The listing builds one solid part. Answer for the finished solid, in the listing's coordinates (mm). A direction names the side the tool comes from. Give positions to 0.01 mm unless a question says otherwise; leave off trailing zeros. Order: outer loops, then holes, each group sorted by start corner. A loop starts at its lowest first (then second) coordinate and runs counter-clockwise, first axis right, second up.
```python
from build123d import *

# Parameters (mm, degrees)
EXTRUDE_1_DEPTH = 4.2
SKETCH_2_R      = 3.5
EXTRUDE_2_DEPTH = 2.1
SKETCH_3_R      = 2.25
EXTRUDE_3_DEPTH = 2
EXTRUDE_START   = -9
EXTRUDE_4_DEPTH = 7


with BuildPart() as part:
    # 草图1 → 凸台-拉伸1 (new body)
    with BuildSketch(Plane.XY):
        with BuildLine():
            ThreePointArc((-6.25, 3.3e-08), (-5.817755734, -2.236089463), (-4.583301282, -4.15))
            Line((-4.583301282, -4.15), (4.583301282, -4.15))
            ThreePointArc((4.583301282, -4.15), (5.817755724, -2.236089488), (6.25, -2.1e-08))
            ThreePointArc((6.25, -2.1e-08), (5.817755732, 2.236089469), (4.583301282, 4.15))
            Line((4.583301282, 4.15), (-4.583301282, 4.15))
            ThreePointArc((-4.583301282, 4.15), (-5.817755722, 2.236089494), (-6.25, 3.3e-08))
        make_face()
    extrude(amount=EXTRUDE_1_DEPTH)

    # 草图2 → 凸台-拉伸2 (add)
    with BuildSketch(Plane.XY.offset(4.2)):
        Circle(SKETCH_2_R)
    extrude(amount=EXTRUDE_2_DEPTH)

    # 草图3 → 凸台-拉伸3 (add)
    with BuildSketch(Plane.XY.offset(6.3)):
        Circle(SKETCH_3_R)
    extrude(amount=EXTRUDE_3_DEPTH)

    # 草图4 → 凸台-拉伸4 (add)
    with BuildSketch(Plane.XY.offset(4.2).offset(EXTRUDE_START)):
        with BuildLine():
            ThreePointArc((-5.812148865, -2.25), (-6.25, 0), (-5.812148865, 2.25))
            Line((-5.812148865, 2.25), (-7, 2.25))
            Line((-7, 2.25), (-7, -2.25))
            Line((-7, -2.25), (-5.812148865, -2.25))
        make_face()
        with BuildLine():
            Line((7, 2.25), (5.812148865, 2.25))
            ThreePointArc((5.812148865, 2.25), (6.25, 0), (5.812148865, -2.25))
            Line((5.812148865, -2.25), (7, -2.25))
            Line((7, -2.25), (7, 2.25))
        make_face()
    extrude(amount=EXTRUDE_4_DEPTH)


solid = part.part
```
1) Find section B-B (x = 0). Write down the section's boundary in (y, z), then the cut area to 3 significant figures.
Geometry says:
outline: (-4.15, 0) - (4.15, 0) - (4.15, 4.2) - (3.5, 4.2) - (3.5, 6.3) - (2.25, 6.3) - (2.25, 8.3) - (-2.25, 8.3) - (-2.25, 6.3) - (-3.5, 6.3) - (-3.5, 4.2) - (-4.15, 4.2) - close
area: 58.6 mm2
2) Find section D-D (z = 4.5). Write down the section's boundary in (x, y).
Geometry says:
outline: circle Ø7 at (0, 0)
3) Straight lines are drawn through the part: probe 1 along Z at (x, y) = (2.75, 2.5); probe 2 along Z at (x, y) = (1, -3.25); probe 3 along X at (y, z) = (0.5, -2.75). For each, find the intervals that lie inside material, in ascending order.
Geometry says:
probe 1: z = 0 to 4.2
probe 2: z = 0 to 6.3
probe 3: x = -7 to -6.23, 6.23 to 7
4) A tool of negligible diameter and unlimited length cuts with its end or side. For faces 5 (the flat face through (-6, -2.25, -1)), 6 (the flat face through (-6, 2.25, -1)), 7 (the flat face through (0, -4, 4.2)), 8 (the flat face through (6, -2.25, -1)), 9 (the cylindrical face through (-6.25, -0.03, -2.43)), from which of +Z, -Z, +X, -X, +Y, -Y can it reach the whole face along a straight path? Write none if from no direction.
Geometry says:
face 5: +Z, -Z, -X, -Y
face 6: +Z, -Z, -X, +Y
face 7: +Z
face 8: +Z, -Z, +X, -Y
face 9: -Z
5) Find section C-C (y = -1.25). Write down the section's boundary in (x, z).
Geometry says:
outline: (-7, -4.8) - (-6.12, -4.8) - (-6.12, 0) - (6.12, 0) - (6.12, -4.8) - (7, -4.8) - (7, 2.2) - (6.12, 2.2) - (6.12, 4.2) - (3.27, 4.2) - (3.27, 6.3) - (1.87, 6.3) - (1.87, 8.3) - (-1.87, 8.3) - (-1.87, 6.3) - (-3.27, 6.3) - (-3.27, 4.2) - (-6.12, 4.2) - (-6.12, 2.2) - (-7, 2.2) - close
6) For a pull along Y with two mould halves and no side action, classify faces 1 (the flat face through (7, 0, -1)), 2 (the cylindrical face through (6.25, 0.03, -2.43)), 3 (the flat face through (6, 2.25, -1)), 4 (the cylindrical face through (3.233, -1.341, 5.235)) as +Y half, -Y half, draft (parallel to the pull), parting line (faces both ways), or undercut.
Geometry says:
face 1: draft
face 2: undercut
face 3: +Y half
face 4: parting line
7) Given P1, Ø2.5, axis at x = -2.5, y = -0.5, coming from the -Z side; P2, Ø1, axis at x = 6.5, z = -1.5, coming from the -Y side; P3, Ø1, axis at x = -6.5, z = -3, coming from the +Y side, each flat-ended and moving along its own axis, determine where each tip first touches the part or whether it passes through.
Geometry says:
P1: stops at z = 0
P2: stops at y = -2.25
P3: stops at y = 2.25
8) Find section A-A (z = -0.75). Write down the section's boundary in (x, y), then the cut area to 3 significant figures.
Geometry says:
outline: (-7, -2.25) - (-5.81, -2.25) arc R6 cw to (-5.81, 2.25) - (-7, 2.25) - close; (5.81, -2.25) - (7, -2.25) - (7, 2.25) - (5.81, 2.25) arc R6 cw to start
area: 8.04 mm2
